Can you work these out from the drawing? Everything is in mm from the part's minimum corner. Give positions to 0.01 mm unless a question says otherwise; leave off trailing zeros. Loops run counter-clockwise (first coordinate to the right, second up) from the corner with the lowest first, then second, coordinate; pieces in that order, holes last. Notation, with made-up numbers: M 25.5,-24 L 77.5,-24 A13 ccw 77.5,-12 Z; hole C 58,-3.75 d3. An arc over 180 degrees is marked long. Use CSV: the item, a comma, the result in double quotes.
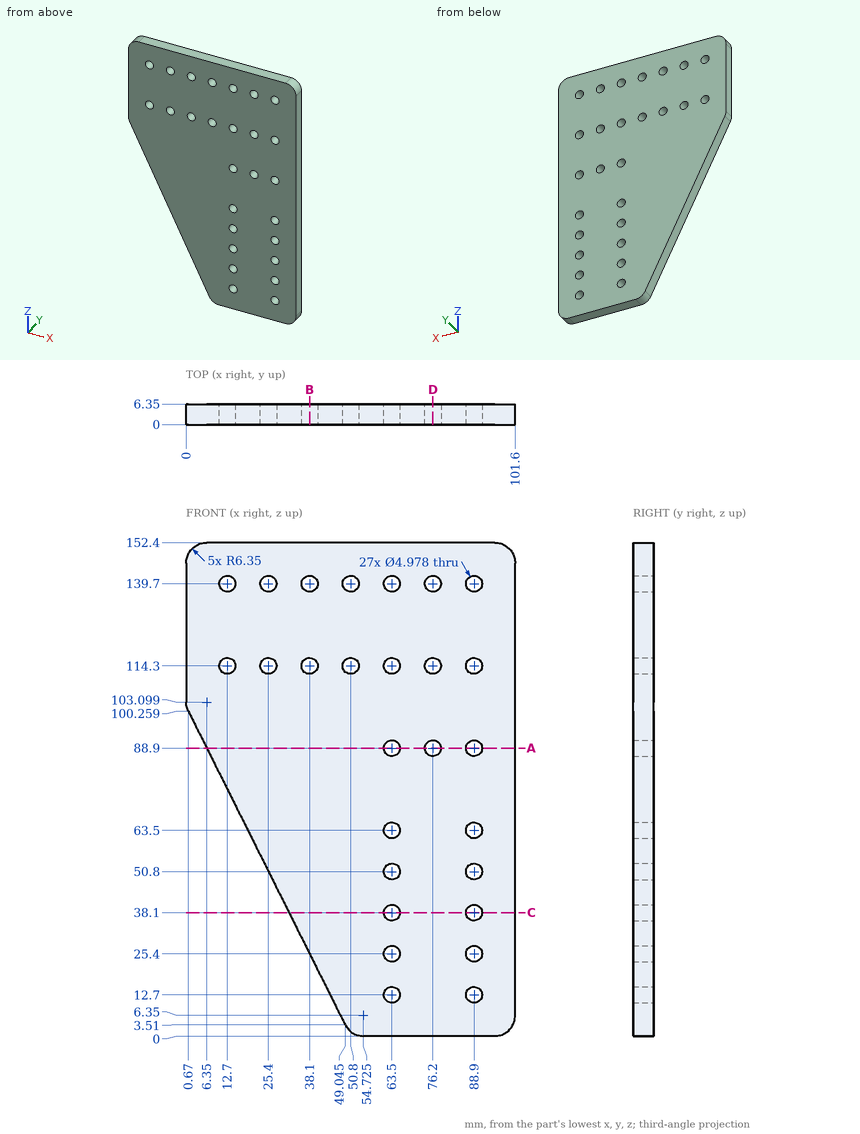
Q1. I want a section at C-C, the plane z = 38.1. Please give me the cut outline in (x, y).
Model answer:
outline,"M 31.75,0 L 61.01,0 L 61.01,6.35 L 31.75,6.35 Z; M 65.99,0 L 86.41,0 L 86.41,6.35 L 65.99,6.35 Z; M 91.39,0 L 101.6,0 L 101.6,6.35 L 91.39,6.35 Z"
Q2. I want a section at A-A, the plane z = 88.9. Please give me the cut outline in (x, y), then the cut area to 3 significant figures.
Model answer:
outline,"M 6.35,0 L 61.01,0 L 61.01,6.35 L 6.35,6.35 Z; M 65.99,0 L 73.71,0 L 73.71,6.35 L 65.99,6.35 Z; M 78.69,0 L 86.41,0 L 86.41,6.35 L 78.69,6.35 Z; M 91.39,0 L 101.6,0 L 101.6,6.35 L 91.39,6.35 Z"
area,"510 mm2"
Q3. I want a section at D-D, the plane x = 76.2. Please give me the cut outline in (y, z).
Model answer:
outline,"M 0,0 L 6.35,0 L 6.35,86.41 L 0,86.41 Z; M 0,91.39 L 6.35,91.39 L 6.35,111.81 L 0,111.81 Z; M 0,116.79 L 6.35,116.79 L 6.35,137.21 L 0,137.21 Z; M 0,142.19 L 6.35,142.19 L 6.35,152.4 L 0,152.4 Z"
Q4. Please list where these lines run through material, in increasing order: L1, parallel to Z at x = 76.2, y = 3.5; L2, parallel to Z at x = 50.8, y = 3.75; L3, parallel to Z at x = 12.7, y = 2.75 (1 decimal). Write a range as from..to.
Model answer:
L1,"0..86.41, 91.39..111.81, 116.79..137.21, 142.19..152.4"
L2,"1.36..111.81, 116.79..137.21, 142.19..152.4"
L3,"76.2..111.8, 116.8..137.2, 142.2..152.4"
Q5. I want a section at B-B, the plane x = 38.1. Please give me the cut outline in (y, z), then the cut area to 3 significant figures.
Model answer:
outline,"M 0,25.4 L 6.35,25.4 L 6.35,111.81 L 0,111.81 Z; M 0,116.79 L 6.35,116.79 L 6.35,137.21 L 0,137.21 Z; M 0,142.19 L 6.35,142.19 L 6.35,152.4 L 0,152.4 Z"
area,"743 mm2"
